Verification items for this drawing (mm, ordinates from the low corner). Give positions to 0.01 mm unless a question says otherwise; leave off trailing zeros. Loops run counter-clockwise (first coordinate to the right, second up) from the corner with the lowest first, then second, coordinate; pieces in that order, holes last. Notation, with made-up numbers: (-18, 87.25) - (3, 87.25) arc R19 cw to (3, 110.25) - close; hole circle Ø1 at (20, 9). An arc over 180 degrees is marked (long way). Write item = value, one per line. Start each with the question number.
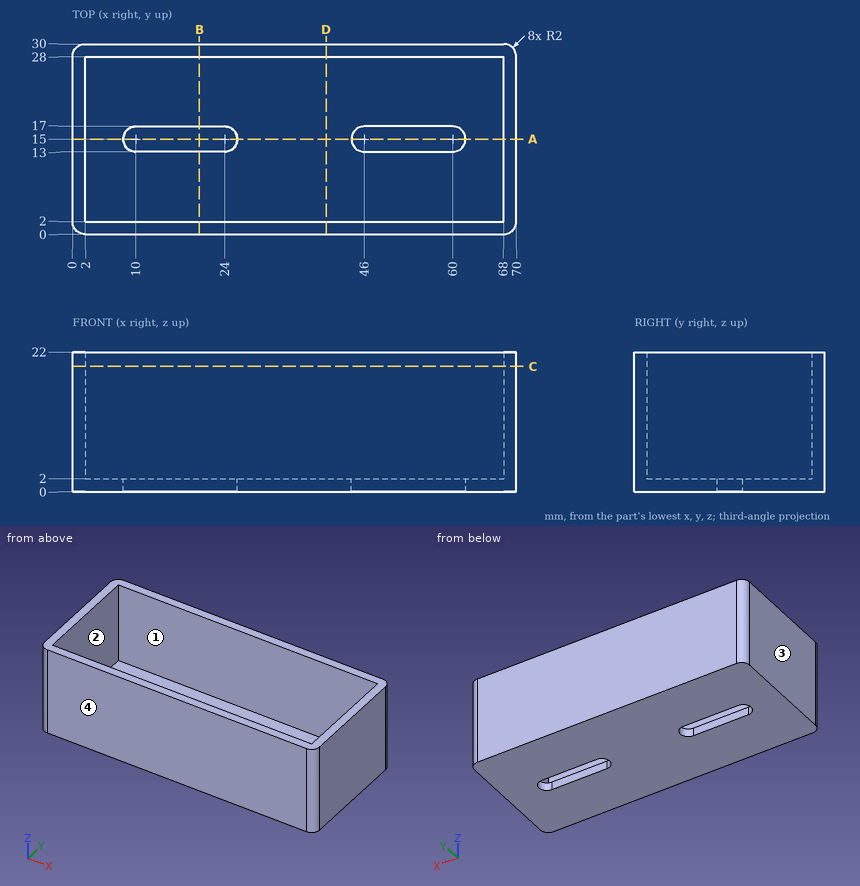
1) Cross-section at C-C on z = 19.75. Enter the section's corners in (x, y), and give its area (3 significant figures).
2) Cross-section at B-B on x = 20. Enter the section's corners in (y, z).
3) Material ranges on line 1 along X through (y, z) = (19, 4); line 2 along Y through (x, z) = (41, 17.25); line 3 along Y through (x, z) = (47.5, 1.5), recorded low to high.
4) Gauge pin test, flat end, axial feed: P1, Ø8, axis at x = 42, y = 10.5, coming from the +Z side. Record the tip position at first contact, or that the pin passes through.
5) Release check for a two-part mould opening along X. For the marked faces 1, 2, 3 and 4 record: pulls with the +X half, pulls with the -X half, needs draft (parallel to the pull), parting line crosses it, or undercut.
6) Cross-section at D-D on x = 40. Enter the section's corners in (y, z).
7) Cross-section at A-A on y = 15. Enter the section's corners in (x, z), and give its area (3 significant figures).
Checked values:
q1.outline = (0, 2) arc R2 ccw to (2, 0) - (68, 0) arc R2 ccw to (70, 2) - (70, 28) arc R2 ccw to (68, 30) - (2, 30) arc R2 ccw to (0, 28) - close; hole (2, 2) - (68, 2) - (68, 28) - (2, 28) - close
q1.area = 381 mm²
q2.outline = (0, 0) - (13, 0) - (13, 2) - (2, 2) - (2, 22) - (0, 22) - close; (17, 0) - (30, 0) - (30, 22) - (28, 22) - (28, 2) - (17, 2) - close
q3.line_1 = 0 to 2, 68 to 70
q3.line_2 = 0 to 2, 28 to 30
q3.line_3 = 0 to 13, 17 to 30
q4.P1 = 2
q5.face_1 = undercut
q5.face_2 = undercut
q5.face_3 = pulls with the -X half
q5.face_4 = needs draft
q6.outline = (0, 0) - (30, 0) - (30, 22) - (28, 22) - (28, 2) - (2, 2) - (2, 22) - (0, 22) - close
q7.outline = (0, 0) - (8, 0) - (8, 2) - (2, 2) - (2, 22) - (0, 22) - close; (26, 0) - (44, 0) - (44, 2) - (26, 2) - close; (62, 0) - (70, 0) - (70, 22) - (68, 22) - (68, 2) - (62, 2) - close
q7.area = 148 mm²
